Drawing for the job (mm, zero at the part's lowest x, y, z). Give positions to 0.01 mm unless a question says otherwise; leave off trailing zeros. Loops run counter-clockwise (first coordinate to the right, second up) from the corner with the lowest first, then second, coordinate; pieces in that order, holes last. Notation, with made-up numbers: (13.5, 55) -> (56.5, 55) arc R17 cw to (56.5, 85) -> close; hole circle Ø2 at (57.5, 46.5). An arc over 180 degrees is marked (long way). Write item = value, one per line.
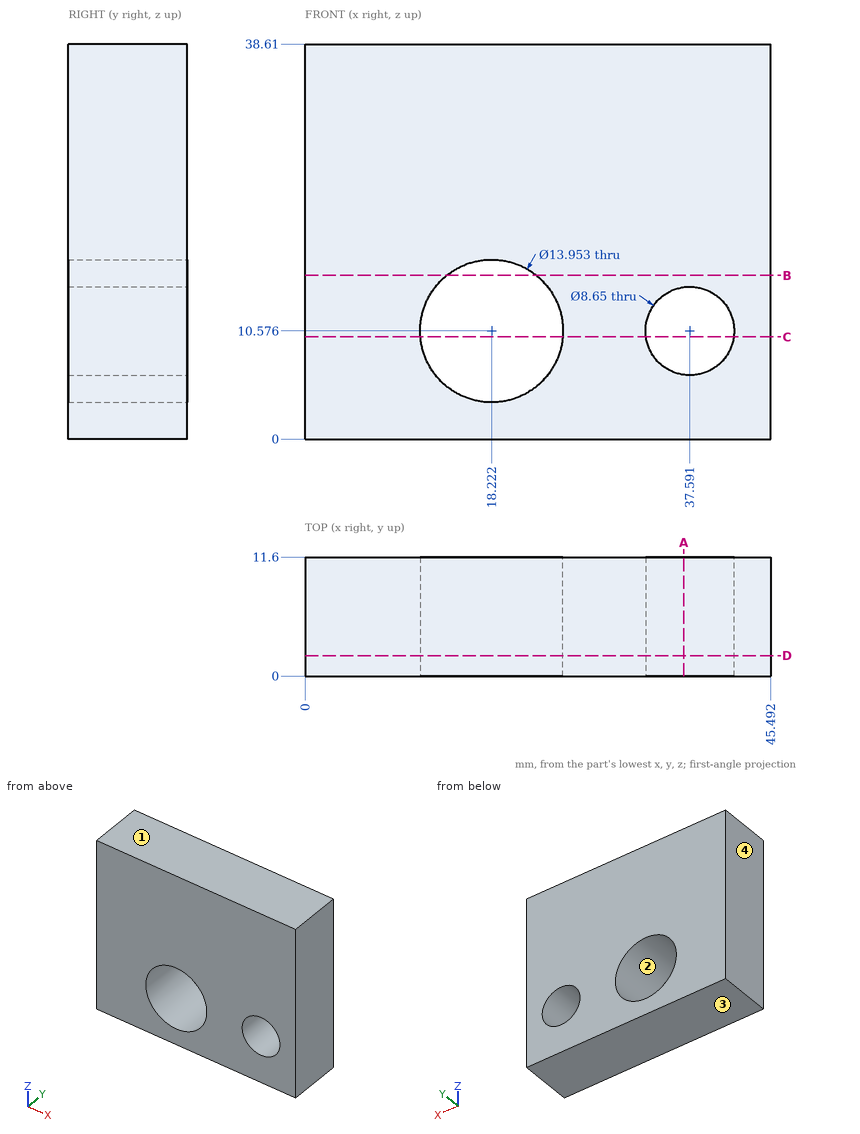
1) Pull direction Z, two halves, no side cores. Call the marked faces 1, 2, 3 and 4: pulls with the +Z half, pulls with the -Z half, needs draft (parallel to the pull), parting line crosses it, or undercut.
Resolved:
face_1 = pulls with the +Z half
face_2 = undercut
face_3 = pulls with the -Z half
face_4 = needs draft
2) Slice it at A-A, the plane x = 37. List the corners of the cut face in (y, z).
Resolved:
outline = (0, 0) -> (11.6, 0) -> (11.6, 6.29) -> (0, 6.29) -> close; (0, 14.86) -> (11.6, 14.86) -> (11.6, 38.61) -> (0, 38.61) -> close
3) Slice it at B-B, the plane z = 16. List the corners of the cut face in (x, y).
Resolved:
outline = (0, 0) -> (13.83, 0) -> (13.83, 11.6) -> (0, 11.6) -> close; (22.61, 0) -> (45.49, 0) -> (45.49, 11.6) -> (22.61, 11.6) -> close
4) Slice it at C-C, the plane z = 10. List the corners of the cut face in (x, y) (1 decimal), and give its area (3 significant figures).
Resolved:
outline = (0, 0) -> (11.3, 0) -> (11.3, 11.6) -> (0, 11.6) -> close; (25.2, 0) -> (33.3, 0) -> (33.3, 11.6) -> (25.2, 11.6) -> close; (41.9, 0) -> (45.5, 0) -> (45.5, 11.6) -> (41.9, 11.6) -> close
area = 267 mm²
5) Drill centre lines: line 1 along X through (y, z) = (11.25, 11) (1 decimal); line 2 along X through (y, z) = (1, 8) (1 decimal); line 3 along Z through (x, y) = (18, 2). Where is each one in solid material? Low to high. Write a range as [from, to].
Resolved:
line_1 = [0, 11.3], [25.2, 33.3], [41.9, 45.5]
line_2 = [0, 11.7], [24.7, 34.1], [41.1, 45.5]
line_3 = [0, 3.6], [17.55, 38.61]
6) Slice it at D-D, the plane y = 2. Count the separate pieces of the cut face and the enclosed holes in it, and give its area (4 significant figures).
Resolved:
separate_pieces = 1
enclosed_holes = 2
area = 1,545 mm²
